CAD build for the part. Positions are in the model's coordinates, mm. Face numbers are marked on the shaded views. A direction names the side the tool comes from. Round coordinates to 2 decimals unless told otherwise and drop trailing zeros. Loops run counter-clockwise (first coordinate to the right, second up) from the corner with the lowest first, then second, coordinate; pieces in that order, holes last. Notation, with made-up numbers: M 76.5,62 L 81.5,62 A35 ccw 81.5,96 Z; hole C 20,76 d2. An arc over 180 degrees is marked long. Use a Markdown table: item, result. Add a question column.
(1) Band-saw the part on D-D, the plane y = 3.25. Write the cut outline in (x, z).
(2) Band-saw the part on A-A, the plane z = 0. Write the cut outline in (x, y).
(3) Wall check: L1, parallel to X at y = 0.25, z = 0; L2, parallel to X at y = -0.75, z = -1.5; L3, parallel to Z at x = 42.5, y = 1.25. Give the ranges that are in metal, low to high.
(4) Band-saw the part on C-C, the plane x = 53.5. Write the cut outline in (y, z), and give its area (3 significant figures).
(5) Flat gauge pins, fed straight in: P1, Ø2, axis at x = 34.5, y = -1, coming from the -Z side; P2, Ø1.5, axis at y = -2, z = -2.5, coming from the +X side; P3, Ø1.5, axis at y = -1, z = 6, coming from the +X side. Where does each tip first touch, or does it go through?
(6) Which spindle directions (+Z, -Z, +X, -X, +Y, -Y) get a long thin tool onto all of the face, cutting with end or side? Do the marked faces 1 and 2. Say none if no direction does.
(7) Band-saw the part on B-B, the plane y = 0. Write the cut outline in (x, z), and give its area (3 significant figures).
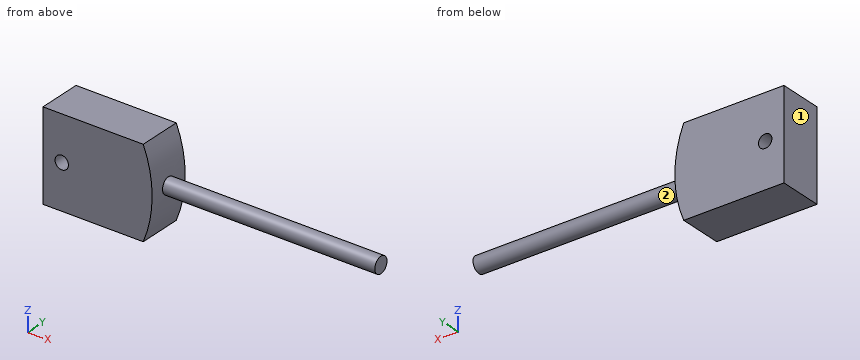
from build123d import *

# Parameters (mm, degrees)
BOSS_EXTRUDE1_DEPTH      = 4.1275
BOSS_EXTRUDE1_DEPTH_BACK = 4.1275
SKETCH1_R                = 1.27


with BuildPart() as part:
    # Sketch1 → Boss-Extrude1 (new, two sides: drawn at the far end of the back side and taken through both)
    with BuildSketch(Plane(origin=(0, 0, 0), x_dir=(1, 0, 0), z_dir=(0, 1, 0)).offset(-BOSS_EXTRUDE1_DEPTH_BACK)):
        with BuildLine():
            Line((0, 8.4582), (19.010911587, 8.4582))
            ThreePointArc((19.010911587, 8.4582), (20.701, 0), (19.010911587, -8.4582))
            Line((19.010911587, -8.4582), (0, -8.4582))
            Line((0, -8.4582), (0, 8.4582))
        make_face()
        with Locations(Location((3.556, 0, 0), (0, 0, 270))):
            Circle(SKETCH1_R, mode=Mode.SUBTRACT)
    extrude(amount=BOSS_EXTRUDE1_DEPTH + BOSS_EXTRUDE1_DEPTH_BACK)

    # Sketch2 → Revolve1 (revolve)
    with BuildSketch(Plane(origin=(0, 0, 0), x_dir=(1, 0, 0), z_dir=(0, 1, 0))):
        Polygon((20.701, 0), (60.96, 0), (60.96, 1.524), (20.701, 1.524), (20.016943544, 1.524), (20.016943544, 0), align=None)
    revolve(axis=Axis((21.73605, 0, 0), (-1, 0, 0)))


solid = part.part
Return value:
| question | item | result |
|---|---|---|
| 1 | outline | M 0,-8.46 L 19.01,-8.46 A22.01 ccw 19.01,8.46 L 0,8.46 Z; hole C 3.56,0 d2.54 |
| 2 | outline | M 0,-4.13 L 2.29,-4.13 L 2.29,4.13 L 0,4.13 Z; M 4.83,-4.13 L 20.7,-4.13 L 20.7,-1.52 L 60.96,-1.52 L 60.96,1.52 L 20.7,1.52 L 20.7,4.13 L 4.83,4.13 Z |
| 3 | L1 | 0 to 2.29, 4.83 to 60.96 |
| 3 | L2 | 0 to 20.65 |
| 3 | L3 | -0.87 to 0.87 |
| 4 | outline | C 0,0 d3.05 |
| 4 | area | 7.30 mm^2 |
| 5 | P1 | z = -1.52 |
| 5 | P2 | x = 20.63 |
| 5 | P3 | x = 20.07 |
| 6 | face 1 | +Z, -Z, -X, +Y, -Y |
| 6 | face 2 | +X |
| 7 | outline | M 0,-8.46 L 19.01,-8.46 A22.01 ccw 20.65,-1.52 L 60.96,-1.52 L 60.96,1.52 L 20.65,1.52 A22.01 ccw 19.01,8.46 L 0,8.46 Z; hole C 3.56,0 d2.54 |
| 7 | area | 459 mm^2 |
